```python
from build123d import *

# Parameters (mm, degrees)
SKETCH014_R     = 1.5
POCKET002_DEPTH = 21
PAD010_DEPTH    = 10.5
PAD011_DEPTH    = 12.1
SKETCH046_W     = 0.8
SKETCH046_H     = 0.8
POCKET004_DEPTH = 10.5


with BuildPart() as part:
    # Sketch011 → Revolution004 (revolve)
    with BuildSketch(Plane.XY):
        Polygon((0, -0.4), (0.84, -0.4), (2.52, 1), (5.88, -1.8), (7.56, -0.4), (8.4, -0.4), (8.4, -10.9), (7.56, -10.9), (5.88, -12.3), (2.52, -9.5), (0.84, -10.9), (0, -10.9), align=None)
    revolve(axis=Axis((0, 0, 0), (0, 1, 0)))

    # Sketch014 → Pocket002 (cut)
    with BuildSketch(Plane.XZ.offset(-1)):
        Circle(SKETCH014_R)
    extrude(amount=POCKET002_DEPTH, mode=Mode.SUBTRACT)

    # Sketch025 → Pad010 (join)
    with BuildSketch(Plane.XZ.offset(0.4)):
        with BuildLine():
            Line((-10.08, -0.4), (-10.08, -9.2))
            Line((-10.08, -9.2), (5.939697, -9.2))
            Line((5.939697, -9.2), (5.939697, -5.939697))
            ThreePointArc((-8.390471, -0.4), (-3.028801, -7.834945), (5.939697, -5.939697))
            Line((-8.390471, -0.4), (-10.08, -0.4))
        make_face()
    extrude(amount=PAD010_DEPTH)

    # Sketch026 → Pad011 (join)
    with BuildSketch(Plane.XZ.offset(-0.4)):
        with BuildLine():
            ThreePointArc((6.739697, -6.262307), (8.487687, -3.549531), (9.1913, -0.4))
            Line((9.1913, -0.4), (10.08, -0.4))
            Line((10.08, -0.4), (10.08, -9.2))
            Line((10.08, -9.2), (5.939697, -9.2))
            Line((5.939697, -8.4), (5.939697, -9.2))
            Line((6.739697, -8.4), (5.939697, -8.4))
            Line((6.739697, -8.4), (6.739697, -6.262307))
        make_face()
    extrude(amount=PAD011_DEPTH)

    # Sketch046 → Pocket004 (cut)
    with BuildSketch(Plane.XZ.offset(-0.4)):
        with Locations((6.339697, -8.8)):
            Rectangle(SKETCH046_W, SKETCH046_H)
    extrude(amount=POCKET004_DEPTH, mode=Mode.SUBTRACT)


solid = part.part
```
Could you check a few things on this model? Use its own coordinates, in mm. A direction names the side the tool comes from. Round coordinates to 2 decimals unless told otherwise and drop trailing zeros. Loops run counter-clockwise (first coordinate to the right, second up) from the corner with the lowest first, then second, coordinate; pieces in that order, holes last. Notation, with made-up numbers: (28, 81) -> (41, 81) arc R12 cw to (41, 100) -> close; hole circle Ø1 at (32.25, 44). An arc over 180 degrees is marked (long way). Put each result on its own line as item: value.
Q1. I want a section at B-B on x = 0. Write out the boundary of the cut face in (y, z), and give its area (3 significant figures).
Checks:
outline: (-12.3, -5.88) -> (-10.9, -7.56) -> (-10.9, -9.2) -> (-0.4, -9.2) -> (-0.4, -7.56) -> (-1.8, -5.88) -> (1, -2.52) -> (0.15, -1.5) -> (-10.35, -1.5) -> (-9.5, -2.52) -> close; (-12.3, 5.88) -> (-9.5, 2.52) -> (-10.35, 1.5) -> (0.15, 1.5) -> (1, 2.52) -> (-1.8, 5.88) -> (-0.4, 7.56) -> (-0.4, 8.4) -> (-10.9, 8.4) -> (-10.9, 7.56) -> close
area: 153 mm2
Q2. Please list where these lines run through material, in increasing order: line 1 (X direction, y = -6.75, z = 0); line 2 (X direction, y = -9.5, z = -7.5); line 3 (Z direction, x = 4.25, y = -1.25). Write a range as from..to.
Checks:
line 1: -8.4..-1.5, 1.5..8.4
line 2: -10.08..5.94, 6.74..10.08
line 3: -9.2..-4.97, -3.03..3.03, 4.97..7.25
Q3. Which directions (+Z, -Z, +X, -X, +Y, -Y) give clear straight access to the entire face, cutting with the end or side of a thin tool? Please do faces 1 (the flat face through (10.08, -6, -5)), 2 (the flat face through (-6, -10.9, -5)), 3 (the cylindrical face through (8.47, -5.57, -3.59)), 4 (the flat face through (6.3, -10.1, -8.8)), 5 (the flat face through (0, -6, -9.2)).
Checks:
face 1: +Z, -Z, +X, +Y, -Y
face 2: -Y
face 3: +Y, -Y
face 4: -Z, +Y
face 5: -Z, +X, -X, +Y, -Y
Q4. Thinking about a two-plate mould opening in Z: for faces 6 (the flat face through (9, 0.4, -6)), 7 (the cylindrical face through (-1.5, -5.03, 0.07)), 8 (the conical face through (2.56, -9.64, -0.81)), 9 (the flat face through (-9, -6, -0.4)), which applies, pulls with the +Z half, pulls with the -Z half, needs draft (parallel to the pull), parting line crosses it, or undercut?
Checks:
face 6: needs draft
face 7: undercut
face 8: undercut
face 9: pulls with the +Z half
Q5. I want a section at C-C on z = 0. Write out the boundary of the cut face in (x, y), and give its area (3 significant figures).
Checks:
outline: (-8.4, -10.9) -> (-7.56, -10.9) -> (-5.88, -12.3) -> (-2.52, -9.5) -> (-1.5, -10.35) -> (-1.5, 0.15) -> (-2.52, 1) -> (-5.88, -1.8) -> (-7.56, -0.4) -> (-8.4, -0.4) -> close; (1.5, -10.35) -> (2.52, -9.5) -> (5.88, -12.3) -> (7.56, -10.9) -> (8.4, -10.9) -> (8.4, -0.4) -> (7.56, -0.4) -> (5.88, -1.8) -> (2.52, 1) -> (1.5, 0.15) -> close
area: 145 mm2
Q6. I want a section at A-A on y = -3.5. Write out the boundary of the cut face in (x, z).
Checks:
outline: (-10.08, -9.2) -> (5.94, -9.2) -> (5.94, -5.94) arc R8.4 ccw (long way) to (-8.39, -0.4) -> (-10.08, -0.4) -> close; (6.74, -9.2) -> (10.08, -9.2) -> (10.08, -0.4) -> (9.19, -0.4) arc R9.2 cw to (6.74, -6.26) -> close; hole circle Ø3 at (0, 0)
Q7. For pin 1 Ø0.8 at (x, y) = (-9.5, -8) entering from +Z; pin 2 Ø0.9 at (y, z) = (-11.5, -9) entering from -X; pin 3 Ø1.5 at (x, z) = (7.5, 2) entering from -Y, each with a flat end and sliding along its axis, tell me the tip position at first contact or that it passes through.
Checks:
pin 1: z = -0.4
pin 2: x = 5.94
pin 3: y = -11.36
